Read the model definition and answer for the solid it produces. Units are mm, in the model's axes. Face numbers are marked on the shaded views. Give positions to 0.01 mm unless a question says otherwise; leave off trailing zeros. Order: outer loops, then holes, each group sorted by start corner. A loop starts at its lowest first (then second) coordinate and runs counter-clockwise, first axis right, second up. Notation, with made-up numbers: (59.5, 65) - (104.5, 65) arc R23 cw to (104.5, 82) - close; hole circle Ø9 at (-12, 86.25). An arc over 180 degrees is marked (long way). Return JSON: item names as keys, results as strings.
Autodesk Inventor part; units mm, degrees
ref_plane "YZ Plane" through (0, 0, 0) normal (1, 0, 0) x (0, 1, 0)
ref_plane "XZ Plane" through (0, 0, 0) normal (0, 1, 0) x (-1, 0, 0)
ref_plane "XY Plane" through (0, 0, 0) normal (0, 0, 1) x (1, 0, 0)
sketch "草圖1" plane through (0, 0, 0) normal (1, 0, 0) x (0, 1, 0)
  circle A0 centre (0, 0) radius 15
  dimension "d0" = 30
extrude "擠出1" add sketch "草圖1" along normal mid plane 6
sketch "草圖2" plane through (3, 0, 0) normal (1, 0, 0) x (0, 0, -1)
  circle A0 centre (0, 0) radius 3.5
  dimension "d3" = 7
extrude "擠出2" add sketch "草圖2" along normal blind 68.5
sketch "草圖3" plane through (-3, 0, 0) normal (-1, 0, 0) x (0, 0, 1)
  circle A0 centre (0, 0) radius 3.5
  dimension "d6" = 7
extrude "擠出3" add sketch "草圖3" along normal blind 68.5
sketch "草圖9" plane through (-71.5, 0, 0) normal (-1, 0, 0) x (0, 0, 1)
  circle A0 centre (0, 0) radius 12
  dimension "d27" = 24
extrude "擠出8" add sketch "草圖9" against normal blind 5
sketch "草圖11" plane through (71.5, 0, 0) normal (1, 0, 0) x (0, 0, -1)
  circle A0 centre (0, 0) radius 12
  dimension "d30" = 24
extrude "擠出9" add sketch "草圖11" against normal blind 5
sketch "草圖12" plane through (71.5, 0, 0) normal (1, 0, 0) x (0, 0, -1)
  circle A0 centre (0, -8) radius 2
  circle A1 centre (8, 0) radius 2
  circle A2 centre (0, 8) radius 2
  circle A3 centre (-8, 0) radius 2
  point P0 (0, 0)
  dimension "d33" = 4
  dimension "d36" = 360
extrude "擠出10" cut sketch "草圖12" against normal blind 5
sketch "草圖13" plane through (-71.5, 0, 0) normal (-1, 0, 0) x (0, 0, 1)
  circle A0 centre (0, -8) radius 2
  circle A1 centre (8, 0) radius 2
  circle A2 centre (0, 8) radius 2
  circle A3 centre (-8, 0) radius 2
  point P0 (0, 0)
  dimension "d40" = 4
  dimension "d43" = 360
extrude "擠出11" cut sketch "草圖13" against normal blind 5
properties part number "煞車桿"
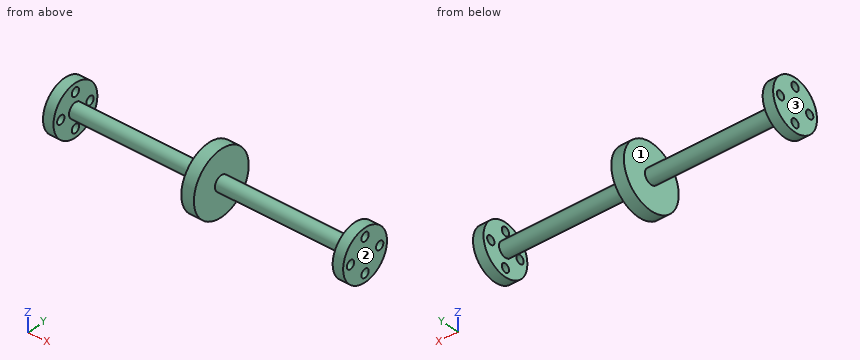
Q1. A cutting plane is placed at A-A (z = 7.25). Write down the section's boundary in (x, y), and give its area (3 significant figures).
Values:
{"outline": "(-71.5, -9.56) - (-66.5, -9.56) - (-66.5, -1.85) - (-71.5, -1.85) - close; (-71.5, 1.85) - (-66.5, 1.85) - (-66.5, 9.56) - (-71.5, 9.56) - close; (-3, -13.13) - (3, -13.13) - (3, 13.13) - (-3, 13.13) - close; (66.5, -9.56) - (71.5, -9.56) - (71.5, -1.85) - (66.5, -1.85) - close; (66.5, 1.85) - (71.5, 1.85) - (71.5, 9.56) - (66.5, 9.56) - close", "area": "312 mm²"}
Q2. A cutting plane is placed at B-B (y = 8). Write down the section's boundary in (x, z).
Values:
{"outline": "(-71.5, -8.94) - (-66.5, -8.94) - (-66.5, -2) - (-71.5, -2) - close; (-71.5, 2) - (-66.5, 2) - (-66.5, 8.94) - (-71.5, 8.94) - close; (-3, -12.69) - (3, -12.69) - (3, 12.69) - (-3, 12.69) - close; (66.5, -8.94) - (71.5, -8.94) - (71.5, -2) - (66.5, -2) - close; (66.5, 2) - (71.5, 2) - (71.5, 8.94) - (66.5, 8.94) - close"}
Q3. Consider L1, parallel to X at y = -4.75, z = -0.5; L2, parallel to Y at x = -68, z = 0; L3, parallel to X at y = 10, z = -10. Determine where each line is inside the solid, lowest interval first.
Values:
{"L1": "x = -71.5 to -66.5, -3 to 3, 66.5 to 71.5", "L2": "y = -12 to -10, -6 to 6, 10 to 12", "L3": "x = -3 to 3"}
Q4. A cutting plane is placed at C-C (x = 7). Write down the section's boundary in (y, z), and give its area (3 significant figures).
Values:
{"outline": "circle Ø7 at (0, 0)", "area": "38.5 mm²"}
Q5. Determine the mould class of the marked faces 1, 2 and 3 for opening direction X: released by +X, released by -X, zero draft, split by the parting line, or undercut.
Values:
{"face 1": "undercut", "face 2": "released by +X", "face 3": "released by -X"}
Q6. Given pin 1 (12 mm diameter, centred on x = 54, y = -4, fed in from -Z); pin 2 (5 mm diameter, centred on x = -36, z = -8, fed in from -Y); pin 3 (2.5 mm diameter, centred on y = 0, z = 8, fed in from +X); pin 4 (10 mm diameter, centred on x = 44.5, z = -4, fed in from -Y), each flat-ended and moving along its own axis, determine where each tip first touches the part or whether it passes through.
Values:
{"pin 1": "stops at z = -3.5", "pin 2": "passes through", "pin 3": "stops at x = 3", "pin 4": "stops at y = -3.5"}
